Source: CAD feature listing. Evaluate the final solid. Frame: model axes, mm. A direction names the side the tool comes from. Round coordinates to 2 decimals unless told otherwise and drop trailing zeros. Write each loop counter-clockwise with the first axis right and the second up, starting at its lowest first coordinate (ties: lowest second). Pieces come first, ordered by that corner, then holes. Notation, with made-up numbers: M -27.75,75.25 L -22.75,75.25 A23 ccw -22.75,85.25 Z; hole C 66.25,7.25 d2. An arc over 180 degrees is marked long. Answer in a Markdown table with one row per item.
from build123d import *

# Parameters (mm, degrees)
F1_DEPTH  = 8
F3_W      = 8
F3_H      = 8
F3_R      = 2.4
F4_DEPTH  = 1.7
F5_R      = 2.4
F6_DEPTH  = 1.7
F11_W     = 18.3417219669
F11_H     = 18.5978962108
F12_DEPTH = 8.001


with BuildPart() as f1:
    # F0 (on Front) → F1 (new body)
    with BuildSketch(Plane.XZ):
        Polygon((-2.4, 9.6), (-4, 9.6), (-4, 0), (4, 0), (4, 9.6), (2.4, 9.6), (2.4, 11.3), (-2.4, 11.3), align=None)
    extrude(amount=F1_DEPTH)

    # F3 (on plane+point) → F4 (cut, through all)
    with BuildSketch(Plane.XY.offset(11.3)):
        with Locations((0, -4)):
            Rectangle(F3_W, F3_H)
        with Locations((0, -4)):
            Circle(F3_R, mode=Mode.SUBTRACT)
    extrude(amount=-F4_DEPTH, mode=Mode.SUBTRACT)

    # F5 (on Top) → F6 (cut)
    with BuildSketch(Plane.XY):
        with Locations((0, -4)):
            Circle(F5_R)
    extrude(amount=F6_DEPTH, mode=Mode.SUBTRACT)

    # F8: F1 across plane


with BuildPart() as f1_1:
    add(f1.part)
    add(f1.part.mirror(Plane.YZ.offset(4)))

    # F10: F1 across plane


with BuildPart() as f1_2:
    add(f1_1.part)
    add(f1_1.part.mirror(Plane.YZ.offset(12)))

    # F11 (on face) → F12 (cut)
    with BuildSketch(Plane.YZ.offset(28)):
        with Locations((-4.3679764494, 6.4113480039)):
            Rectangle(F11_W, F11_H)
    extrude(amount=-F12_DEPTH, mode=Mode.SUBTRACT)


solid = f1_2.part
Q1. Pull-direction query (X, two-part tool) for faces 1 (the flat face through (8, -4, 11.3)), 2 (the flat face through (-4, -4, 5)), 3 (the cylindrical face through (10.398, -3.894, 10.462)), 4 (the cylindrical face through (1.29, -1.976, 0.838)); classes: pulls with the +X half, pulls with the -X half, needs draft (parallel to the pull), parting line crosses it, or undercut.
Solutions:
| item | result |
|---|---|
| face 1 | needs draft |
| face 2 | pulls with the -X half |
| face 3 | undercut |
| face 4 | undercut |
Q2. Section C-C (x = 0.25). Return loops of the section in (y, z).
Solutions:
| item | result |
|---|---|
| outline | M -8,0 L -6.39,0 L -6.39,1.7 L -1.61,1.7 L -1.61,0 L 0,0 L 0,9.6 L -1.61,9.6 L -1.61,11.3 L -6.39,11.3 L -6.39,9.6 L -8,9.6 Z |
Q3. Access query for faces 5 (the cylindrical face through (1.29, -1.976, 10.462)), 6 (the flat face through (8, -8, 5)), 7 (the cylindrical face through (13.602, -3.894, 0.838)). Directions: +Z, -Z, +X, -X, +Y, -Y. A direction counts if a zero-diameter tool reaches every point of the face in a straight line with its end or side. Return the directions, or none.
Solutions:
| item | result |
|---|---|
| face 5 | +Z |
| face 6 | +Z, -Z, +X, -X, -Y |
| face 7 | -Z |
Q4. Contact query for a flat-ended pin moving along its axis: pin 1 Ø4 at (x, y) = (0, -4) entering from -Z. Output: stop coordinate, or through.
Solutions:
| item | result |
|---|---|
| pin 1 | stops at z = 1.7 |
Q5. Section A-A (y = -4). Return loops of the section in (x, z).
Solutions:
| item | result |
|---|---|
| outline | M -4,0 L -2.4,0 L -2.4,1.7 L 2.4,1.7 L 2.4,0 L 5.6,0 L 5.6,1.7 L 10.4,1.7 L 10.4,0 L 13.6,0 L 13.6,1.7 L 18.4,1.7 L 18.4,0 L 20,0 L 20,9.6 L 18.4,9.6 L 18.4,11.3 L 13.6,11.3 L 13.6,9.6 L 10.4,9.6 L 10.4,11.3 L 5.6,11.3 L 5.6,9.6 L 2.4,9.6 L 2.4,11.3 L -2.4,11.3 L -2.4,9.6 L -4,9.6 Z |
Q6. Section B-B (z = 10.25). Return loops of the section in (x, y).
Solutions:
| item | result |
|---|---|
| outline | C 0,-4 d4.8; C 8,-4 d4.8; C 16,-4 d4.8 |
Q7. Material intervals for probe 1 along Y at (x, z) = (16, 0.7); probe 2 along Z at (x, y) = (11, -6.5); probe 3 along X at (y, z) = (-5.5, 1.25), sorted ascending.
Solutions:
| item | result |
|---|---|
| probe 1 | y = -8 to -6.4, -1.6 to 0 |
| probe 2 | z = 0 to 9.6 |
| probe 3 | x = -4 to -1.87, 1.87 to 6.13, 9.87 to 14.13, 17.87 to 20 |
